```python
from build123d import *

# Parameters (mm, degrees)
F0_W      = 85.09
F0_H      = 90.2716
F1_DEPTH  = 11.557
F2_W      = 49.060036246
F2_H      = 59.944
F3_DEPTH  = 59.4614
F4_R      = 20.32
F4_R_2    = 15.875
F5_DEPTH  = 16.51
F4_R_3    = 3.175
F6_DEPTH  = 25.4
F7_DEPTH  = 44.577
F8_R      = 2.3368
F9_DEPTH  = 25.4
F10_DEPTH = 15.1638


with BuildPart() as f1:
    # F0 (on Top) → F1 (new body)
    with BuildSketch(Plane.XY):
        Rectangle(F0_W, F0_H)
    extrude(amount=F1_DEPTH)

    # F2 (on face) → F3 (join)
    with BuildSketch(Plane(origin=(0, 0, 0), x_dir=(1, 0, 0), z_dir=(0, 0, -1))):
        Rectangle(F2_W, F2_H)
    extrude(amount=F3_DEPTH)

    # F4 (on face) → F5 (join)
    with BuildSketch(Plane.XZ.offset(29.972)):
        with Locations((0, -25.9842)):
            Circle(F4_R)
        with Locations((0, -25.9842)):
            Circle(F4_R_2, mode=Mode.SUBTRACT)
    extrude(amount=F5_DEPTH)

    # F4 (on face) → F6 (join)
    with BuildSketch(Plane.XZ.offset(29.972)):
        with Locations((0, -25.9842)):
            Circle(F4_R_2)
        with Locations((0, -25.9842)):
            Circle(F4_R_3, mode=Mode.SUBTRACT)
    extrude(amount=F6_DEPTH)

    # F4 (on face) → F7 (join)
    with BuildSketch(Plane.XZ.offset(29.972)):
        with Locations((0, -25.9842)):
            Circle(F4_R_3)
    extrude(amount=F7_DEPTH)

    # F8 (on face) → F9 (cut)
    with BuildSketch(Plane.XZ.offset(45.1358)):
        with Locations((-18.796, 5.7785)):
            Circle(F8_R)
        with Locations((18.796, 5.7785)):
            Circle(F8_R)
    extrude(amount=-F9_DEPTH, mode=Mode.SUBTRACT)

    # F10 (add, through all): a face of the model
    f10_faces = [f1.faces().sort_by_distance(p)[0] for p in [
        (0, 29.972, -29.7307),
    ]]
    extrude(f10_faces, amount=F10_DEPTH)


solid = f1.part
```
Check sheet for the modelled part. Datum: model origin and axes. Units: mm. A direction names the side the tool comes from. Round coordinates to 2 decimals unless told otherwise and drop trailing zeros. Write each loop counter-clockwise with the first axis right and the second up, starting at its lowest first coordinate (ties: lowest second). Pieces come first, ordered by that corner, then holes. Notation, with made-up numbers: (87, 82) -> (114, 82) arc R23 ccw to (114, 105) -> close; hole circle Ø8 at (68, -32.5). An arc over 180 degrees is marked (long way). Put each result on its own line as item: value.
(1) Sectioned sample at D-D (x = -34). Enter the section's corners in (y, z), plus the area to 3 significant figures.
Values found:
outline: (-45.14, 0) -> (45.14, 0) -> (45.14, 11.56) -> (-45.14, 11.56) -> close
area: 1,040 mm^2
(2) Sectioned sample at B-B (y = -12.5). Enter the section's corners in (x, z) (3 decimals), plus the area to 3 significant figures.
Values found:
outline: (-42.545, 0) -> (-24.53, 0) -> (-24.53, -59.461) -> (24.53, -59.461) -> (24.53, 0) -> (42.545, 0) -> (42.545, 11.557) -> (-42.545, 11.557) -> close
area: 3,900 mm^2
(3) Mould release check, pull along Z, two halves, no side actions. Record for faces 1 (the face through (-1, 1, 11.557)), 2 (the face through (-29, 1, 0)), 3 (the face through (-42.545, -1, 6)): released by +Z, released by -Z, zero draft, split by the parting line, or undercut.
Values found:
face 1: released by +Z
face 2: undercut
face 3: zero draft
(4) Tool access check on faces 4 (the face through (-2.067, -50.865, -10.244)), 5 (the face through (-1, -45.136, 6)), 6 (the face through (42.545, -1, 6)), 7 (the face through (0, -74.549, -26)), 8 (the face through (-24.53, 7, -29)). Record the directions out of +Z, -Z, +X, -X, +Y, -Y that give a thin tool (end or side, any length) a straight path to the whole face; none if there is none.
Values found:
face 4: -Y
face 5: +Z, +X, -X, -Y
face 6: +Z, -Z, +X, +Y, -Y
face 7: +Z, -Z, +X, -X, -Y
face 8: -Z, -X, +Y, -Y
(5) Sectioned sample at A-A (x = 0). Enter the section's corners in (y, z).
Values found:
outline: (-74.55, -29.16) -> (-55.37, -29.16) -> (-55.37, -41.86) -> (-46.48, -41.86) -> (-46.48, -46.3) -> (-29.97, -46.3) -> (-29.97, -59.46) -> (45.14, -59.46) -> (45.14, 11.56) -> (-45.14, 11.56) -> (-45.14, 0) -> (-29.97, 0) -> (-29.97, -5.66) -> (-46.48, -5.66) -> (-46.48, -10.11) -> (-55.37, -10.11) -> (-55.37, -22.81) -> (-74.55, -22.81) -> close
(6) Material ranges on line 1 (Y direction, x = -18, z = 2); line 2 (Y direction, x = 7, z = -9); line 3 (X direction, y = 15, z = -5.5), recorded low to high.
Values found:
line 1: y = -45.14 to 45.14
line 2: y = -46.48 to 45.14
line 3: x = -24.53 to 24.53
(7) Sectioned sample at C-C (z = -18.5). Enter the section's corners in (x, y).
Values found:
outline: (-24.53, -29.97) -> (-18.89, -29.97) -> (-18.89, -46.48) -> (-14, -46.48) -> (-14, -55.37) -> (14, -55.37) -> (14, -46.48) -> (18.89, -46.48) -> (18.89, -29.97) -> (24.53, -29.97) -> (24.53, 45.14) -> (-24.53, 45.14) -> close
(8) Go/stop test with flat-tipped pins: pin 1 Ø6 at (x, y) = (27.5, -35.5) entering from -Z; pin 2 Ø1.4 at (x, z) = (-18, 6.5) entering from -Y; pin 3 Ø1.5 at (x, z) = (-24.5, -52) entering from -Y; pin 4 Ø16 at (x, z) = (-4.5, -25.5) entering from -Y. Record where each tip stops, or that it passes through.
Values found:
pin 1: stops at z = 0
pin 2: stops at y = -19.74
pin 3: stops at y = -29.97
pin 4: stops at y = -74.55
